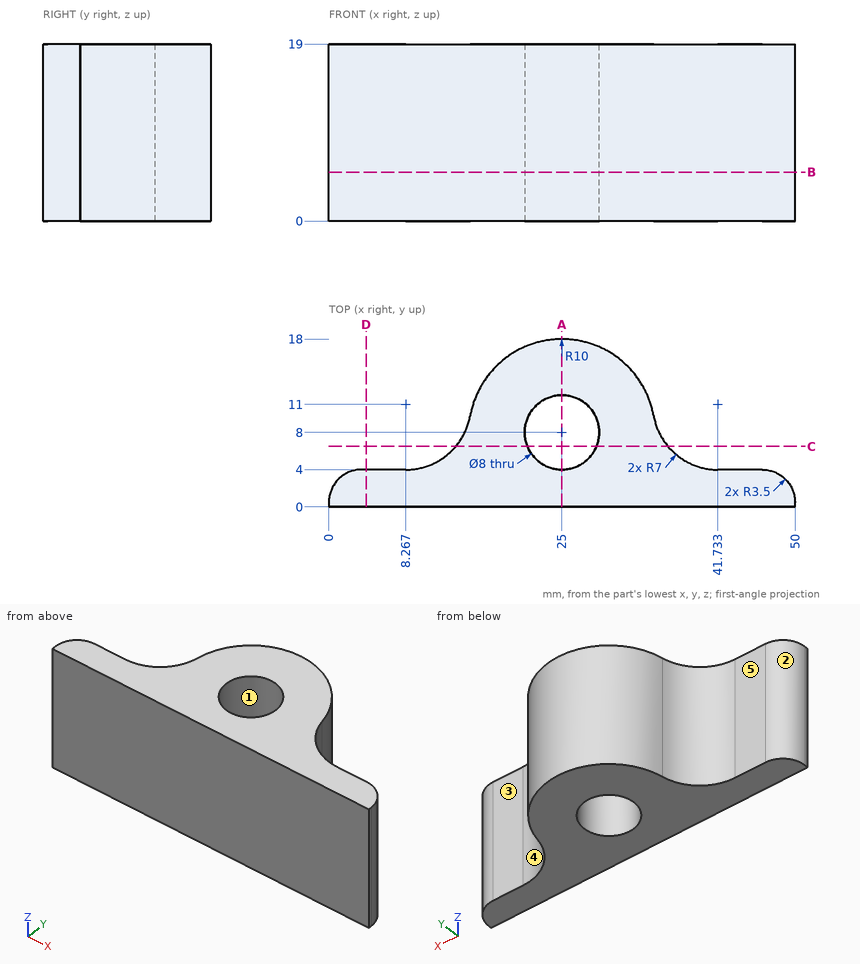
Check sheet for the drawn part. Datum: minimum x, y, z corner. Units: mm. A direction names the side the tool comes from. Round coordinates to 2 decimals unless told otherwise and drop trailing zeros. Order: outer loops, then holes, each group sorted by start corner. A loop starts at its lowest first (then second) coordinate and runs counter-clockwise, first axis right, second up. Notation, with made-up numbers: (87.5, -19) -> (99.5, -19) arc R9 cw to (99.5, -4) -> close; hole circle Ø6 at (64.5, 33.25). An arc over 180 degrees is marked (long way). Put each result on its own line as item: value.
1) Set-up check for the marked faces 4 and 5: record each of +Z, -Z, +X, -X, +Y, -Y from which the full face is reachable in a straight line by a thin tool's end or side.
Final values:
face 4: +Z, -Z, +X, +Y
face 5: +Z, -Z, -X, +Y
2) Mould release check, pull along X, two halves, no side actions. Record for the marked faces 1, 2 and 3: +X half, -X half, draft (parallel to the pull), parting line (faces both ways), or undercut.
Final values:
face 1: undercut
face 2: -X half
face 3: draft
3) Section check B-B (z = 5.25). Record the cut outline in (x, y) (1 decimal).
Final values:
outline: (0, 0) -> (50, 0) -> (50, 0.5) arc R3.5 ccw to (46.5, 4) -> (41.7, 4) arc R7 cw to (34.8, 9.8) arc R10 ccw to (15.2, 9.8) arc R7 cw to (8.3, 4) -> (3.5, 4) arc R3.5 ccw to (0, 0.5) -> close; hole circle Ø8 at (25, 8)
4) Section check A-A (x = 25). Record the cut outline in (y, z).
Final values:
outline: (0, 0) -> (4, 0) -> (4, 19) -> (0, 19) -> close; (12, 0) -> (18, 0) -> (18, 19) -> (12, 19) -> close
5) Section check C-C (y = 6.5). Record the cut outline in (x, z).
Final values:
outline: (13.63, 0) -> (21.29, 0) -> (21.29, 19) -> (13.63, 19) -> close; (28.71, 0) -> (36.37, 0) -> (36.37, 19) -> (28.71, 19) -> close
6) Section check D-D (x = 4). Record the cut outline in (y, z), then the cut area to 3 significant figures.
Final values:
outline: (0, 0) -> (4, 0) -> (4, 19) -> (0, 19) -> close
area: 76.0 mm^2
7) Material ranges on line 1 (Y direction, x = 25, z = 7); line 2 (Y direction, x = 6, z = 9.5); line 3 (Y direction, x = 26.5, z = 3.75), recorded low to high.
Final values:
line 1: y = 0 to 4, 12 to 18
line 2: y = 0 to 4
line 3: y = 0 to 4.29, 11.71 to 17.89
8) Depth check by flat-ended pin: pin 1 (10 mm diameter, centred on y = 6.5, z = 2, fed in from +X); pin 2 (6 mm diameter, centred on y = 8.5, z = 5.5, fed in from -X); pin 3 (1.5 mm diameter, centred on y = 6.5, z = 12, fed in from -X). Enter the tip coordinate at first touch or a pass-through.
Final values:
pin 1: stops at x = 49.85
pin 2: stops at x = 12.6
pin 3: stops at x = 12.9
